```python
from build123d import *

# Parameters (mm, degrees)
F0_W     = 10
F0_H     = 10
F1_DEPTH = 10
F3_D     = 2.7
F4_T     = -1


with BuildPart() as f1:
    # F0 (on Top) → F1 (new body)
    with BuildSketch(Plane.XY):
        with Locations((5, 5)):
            Rectangle(F0_W, F0_H)
    extrude(amount=F1_DEPTH)

    # F3 (through all)
    with Locations(Plane.XY.offset(10)):
        with Locations((5, 5)):
            Hole(F3_D / 2)

    # F4
    f4_openings = [f1.faces().sort_by_distance(p)[0] for p in [
        (0.141421, 5, 10),
    ]]
    offset(amount=F4_T, openings=f4_openings)


solid = f1.part
```
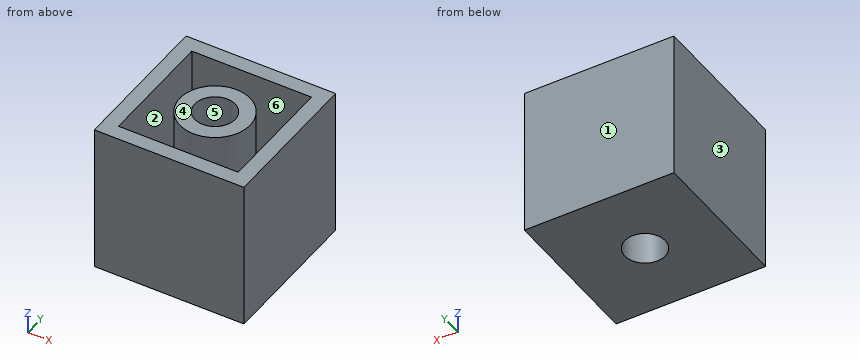
For this review, take the finished solid that the model builds, in its own axes (mm). Face numbers are marked on the shaded views. A direction names the side the tool comes from. Coordinates: 2 decimals unless noted, no trailing zeros. Loops run counter-clockwise (first coordinate to the right, second up) from the corner with the lowest first, then second, coordinate; pieces in that order, holes last. Notation, with made-up numbers: (56, -27) -> (102, -27) arc R27 cw to (102, 1) -> close; hole circle Ø4 at (75, -27). An arc over 180 degrees is marked (long way). Return JSON: item names as keys, results as strings. Group by question number.
(1) Consider section B-B, the plane x = 5. Give the boundary of the cut face in (y, z).
(2) For pin 1 Ø2 at (x, y) = (1.5, 6) entering from -Z, flat-tipped, find the tip position at first contact; note if it passes through.
(3) Mouldability with a two-part tool opening along X and no side actions: class the marked faces 3, 4, 5 and 6 as pulls with the +X half, pulls with the -X half, needs draft (parallel to the pull), parting line crosses it, or undercut.
(4) To check wall thickness, follow L1, parallel to Y at x = 5, z = 7.75; L2, parallel to Y at x = 1.5, z = 7.5. State the ranges of each line that lie inside material, in increasing order.
(5) Consider section A-A, the plane z = 4.25. Give the boundary of the cut face in (x, y), plus the area to 3 significant figures.
(6) Tool access review of the marked faces 1 and 2: name each direction out of +Z, -Z, +X, -X, +Y, -Y from which nothing blocks a thin tool from reaching the whole face with its end or side.
(7) Consider section D-D, the plane x = 1.5. Give the boundary of the cut face in (y, z), plus the area to 3 significant figures.
Results below:
{
 "1": {"outline": "(0, 0) -> (3.65, 0) -> (3.65, 10) -> (2.65, 10) -> (2.65, 1) -> (1, 1) -> (1, 10) -> (0, 10) -> close; (6.35, 0) -> (10, 0) -> (10, 10) -> (9, 10) -> (9, 1) -> (7.35, 1) -> (7.35, 10) -> (6.35, 10) -> close"},
 "2": {"pin 1": "stops at z = 0"},
 "3": {"face 3": "pulls with the -X half", "face 4": "needs draft", "face 5": "undercut", "face 6": "undercut"},
 "4": {"L1": "y = 0 to 1, 2.65 to 3.65, 6.35 to 7.35, 9 to 10", "L2": "y = 0 to 1, 9 to 10"},
 "5": {"outline": "(0, 0) -> (10, 0) -> (10, 10) -> (0, 10) -> close; circle Ø4.7 at (5, 5); hole (1, 1) -> (9, 1) -> (9, 9) -> (1, 9) -> close; hole circle Ø2.7 at (5, 5)", "area": "47.6 mm2"},
 "6": {"face 1": "+Z, -Z, +X, -X, +Y", "face 2": "+Z"},
 "7": {"outline": "(0, 0) -> (10, 0) -> (10, 10) -> (9, 10) -> (9, 1) -> (1, 1) -> (1, 10) -> (0, 10) -> close", "area": "28.0 mm2"}
}
